Verification items for this drawing (mm, ordinates from the low corner). A direction names the side the tool comes from. Coordinates: 2 decimals unless noted, no trailing zeros. Order: outer loops, then holes, each group sorted by start corner. A loop starts at its lowest first (then second) coordinate and runs counter-clockwise, first axis right, second up. Notation, with made-up numbers: M 34.5,-14 L 56.5,-14 A30 cw 56.5,11 Z; hole C 52.5,13.25 d2. An arc over 180 degrees is marked long. Use CSV: the item, a comma, the result in double quotes. Start each with the question number.
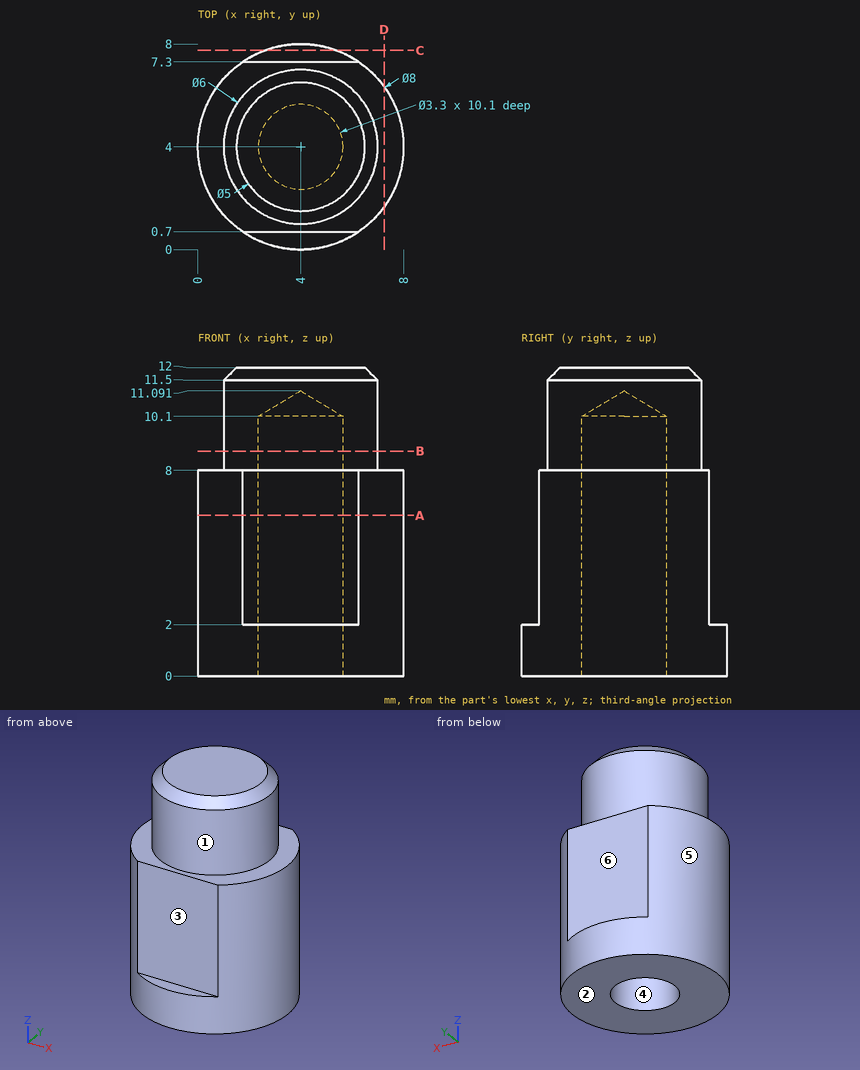
1) Section check B-B on z = 8.75. Record the boundary of the cut face in (x, y).
2) Section check D-D on x = 7.25. Record the boundary of the cut face in (y, z), then the cut area to 3 significant figures.
3) Section check C-C on y = 7.75. Record the boundary of the cut face in (x, z).
4) Gauge pin test, flat ends, axial feed: P1, Ø2.5, axis at x = 4.5, z = 6.5, coming from the +Y side; P2, Ø1.5, axis at y = 7, z = 2, coming from the +X side; P3, Ø1, axis at y = 2, z = 2, coming from the +X side. Record the tip position at first contact, or that the pin passes through.
5) Section check A-A on z = 6.25. Record the boundary of the cut face in (x, y).
6) Material ranges on line 1 along X through (y, z) = (4, 2.5); line 2 along Y through (x, z) = (4, 2.5); line 3 along Z through (x, y) = (0.5, 3.75), recorded low to high.
7) Set-up check for the marked faces 1, 2 and 3: record each of +Z, -Z, +X, -X, +Y, -Y from which the full face is reachable in a straight line by a thin tool's end or side.
8) Draft check along X on the marked faces 4, 5 and 6. Enter one of: +X half, -X half, draft (parallel to the pull), parting line (faces both ways), or undercut.
Results are:
1,outline,"C 4,4 d6; hole C 4,4 d3.3"
2,outline,"M 1.67,0 L 6.33,0 L 6.33,8 L 1.67,8 Z"
2,area,"37.3 mm²"
3,outline,"M 2.61,0 L 5.39,0 L 5.39,2 L 2.61,2 Z"
4,P1,"stops at y = 7.3"
4,P2,"stops at x = 7.31"
4,P3,"stops at x = 7.71"
5,outline,"M 1.74,0.7 L 6.26,0.7 A4 ccw 6.26,7.3 L 1.74,7.3 A4 ccw Z; hole C 4,4 d3.3"
6,line 1,"x = 0 to 2.35, 5.65 to 8"
6,line 2,"y = 0.7 to 2.35, 5.65 to 7.3"
6,line 3,"z = 0 to 8"
7,face 1,"+Z"
7,face 2,"-Z, +X, -X, +Y, -Y"
7,face 3,"+Z, +X, -X, -Y"
8,face 4,"undercut"
8,face 5,"parting line"
8,face 6,"draft"
